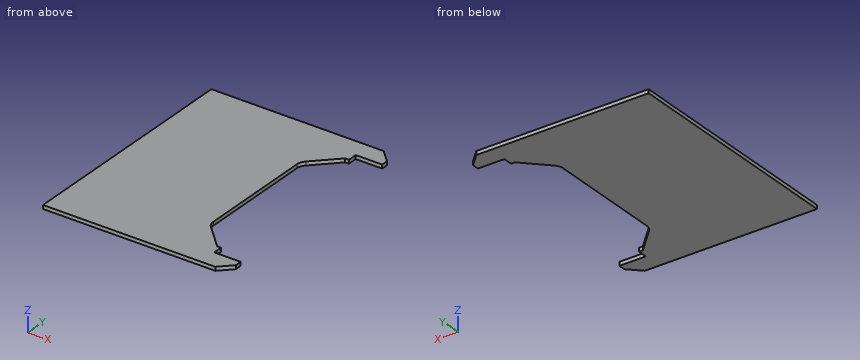
from build123d import *

# Parameters (mm, degrees)
RESSALTO_EXTRUS_O1_DEPTH = 10
CHANFRO1_SIZE            = 70
FILETE1_R                = 30


with BuildPart() as part:
    # Esboço1 → Ressalto-extrusão1 (new body)
    with BuildSketch(Plane.XY):
        Polygon((423, 50), (423, 75), (343, 75), (343, 550), (423, 550), (423, 575), (494, 575), (494, 593), (462, 625), (0, 625), (0, 0), (462, 0), (494, 32), (494, 50), align=None)
    extrude(amount=RESSALTO_EXTRUS_O1_DEPTH)

    # Chanfro1
    chanfro1_edges = [part.edges().sort_by_distance(p)[0] for p in [
        (343, 550, 5),
        (343, 75, 5),
    ]]
    chamfer(chanfro1_edges, length=CHANFRO1_SIZE)

    # Filete1
    filete1_edges = [part.edges().sort_by_distance(p)[0] for p in [
        (343, 145, 5),
        (343, 480, 5),
    ]]
    fillet(filete1_edges, radius=FILETE1_R)


solid = part.part
Geometry: final body of the model. Coordinates: model frame, mm. Round coordinates to 2 decimals unless told otherwise and drop trailing zeros. Order: outer loops, then holes, each group sorted by start corner. A loop starts at its lowest first (then second) coordinate and runs counter-clockwise, first axis right, second up. Notation, with made-up numbers: (53, 5) - (77, 5) arc R24 cw to (77, 18) - close; hole circle Ø2 at (35, 79). An arc over 180 degrees is marked (long way). Write each question's results on one line, items separated by ' | '.
Item 1: First-contact query: pin 1 Ø4 at (x, y) = (216, 440.5) entering from -Z; pin 2 Ø5 at (y, z) = (457.5, 3) entering from +X; pin 3 Ø1 at (y, z) = (80.5, 1.5) entering from +X. Flat tips, straight axial feed; report the tip coordinate or a pass-through.
Completed:
pin 1: z = 0 | pin 2: x = 343 | pin 3: x = 408
Item 2: Section C-C, the plane y = 364. Return the cut outline in (x, z), and give its area (3 significant figures).
Completed:
outline: (0, 0) - (343, 0) - (343, 10) - (0, 10) - close | area: 3,430 mm^2
Item 3: Section D-D, the plane y = 120. Return the cut outline in (x, z).
Completed:
outline: (0, 0) - (368, 0) - (368, 10) - (0, 10) - close
Item 4: Section B-B, the plane z = 8.5. Return the cut outline in (x, y), and give its area (3 significant figures).
Completed:
outline: (0, 0) - (462, 0) - (494, 32) - (494, 50) - (423, 50) - (423, 75) - (413, 75) - (351.79, 136.21) arc R30 cw to (343, 157.43) - (343, 467.57) arc R30 cw to (351.79, 488.79) - (413, 550) - (423, 550) - (423, 575) - (494, 575) - (494, 593) - (462, 625) - (0, 625) - close | area: 237,000 mm^2
Item 5: Material intervals for line 1 along Y through (x, z) = (419, 1); line 2 along Y through (x, z) = (456, 9.5); line 3 along X through (y, z) = (175, 8), sorted ascending. Write a range as [from, to].
Completed:
line 1: [0, 75], [550, 625] | line 2: [0, 50], [575, 625] | line 3: [0, 343]
Item 6: Section A-A, the plane x = 381.5. Return the cut outline in (y, z), and give its area (3 significant figures).
Completed:
outline: (0, 0) - (106.5, 0) - (106.5, 10) - (0, 10) - close; (518.5, 0) - (625, 0) - (625, 10) - (518.5, 10) - close | area: 2,130 mm^2
